Model file for the job. Use its own axes, mm. Face numbers are marked on the shaded views. Coordinates: 2 decimals unless noted, no trailing zeros. Order: outer loops, then holes, each group sorted by start corner. A loop starts at its lowest first (then second) coordinate and runs counter-clockwise, first axis right, second up. Notation, with made-up numbers: (64, -11.5) -> (99, -11.5) arc R13 ccw to (99, -1.5) -> close; hole circle Ø9 at (-8, -17). An arc over 180 degrees is marked (long way). Write item = value, one per line. Start each with the question number.
Q1. Flat gauge pins, fed straight in: pin 1 (8 mm diameter, centred on x = 12.5, y = -11.5, fed in from +Z); pin 2 (10 mm diameter, centred on x = 9.5, z = 22, fed in from +Y); pin 3 (5 mm diameter, centred on x = 11.5, z = 77.5, fed in from +Y); pin 4 (8 mm diameter, centred on y = -5.5, z = 38.5, fed in from -X). Where does each tip first touch, or does it go through?
Q2. Cut at A-A, the plane z = 82.5. List the corners of the cut face in (x, y), plus the area to 3 significant figures.
Q3. Wall check: line 1 (Y direction, x = 5, z = 59.5); line 2 (Z direction, x = -11.5, y = 11); line 3 (X direction, y = 22, z = 76). Give the ranges that are in metal, low to high. Write a range as from..to.
Q4. Cut at B-B, the plane y = 3. List the corners of the cut face in (x, z).
Q5. Cut at D-D, the plane y = -29. List the corners of the cut face in (x, z), plus the area to 3 significant figures.
Q6. Cut at C-C, the plane z = 45.5. List the corners of the cut face in (x, y), plus the area to 3 significant figures.
Q7. Mould opens along Z. For the marked faces 1, 2 and 3 say: +Z half, -Z half, draft (parallel to the pull), parting line (faces both ways), or undercut.
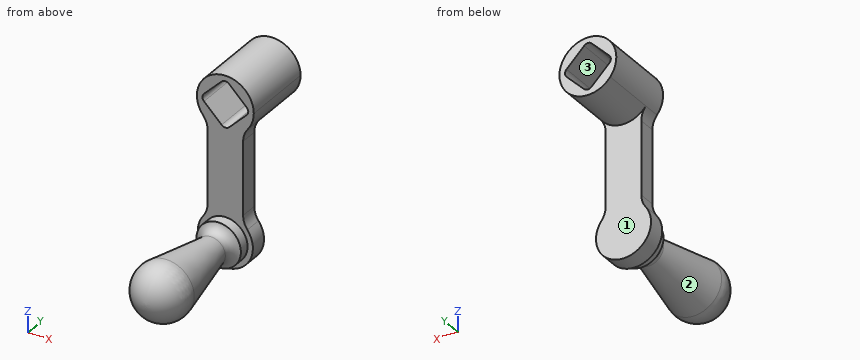
from build123d import *

# Parameters (mm, degrees)
F1_DEPTH = 10
F2_DEPTH = 32


with BuildPart() as f1:
    # F0 (on Front) → F1 (new body)
    with BuildSketch(Plane.XZ):
        with BuildLine():
            ThreePointArc((16, 75), (-5.237229, 90.118579), (-12.571429, 65.102567))
            ThreePointArc((-12.571429, 65.102567), (0, 59), (12.571429, 65.102567))
            ThreePointArc((12.571429, 65.102567), (15.118579, 69.762771), (16, 75))
        make_face()
        with BuildLine():
            Line((2.12132, 87.020815), (12.020815, 77.12132))
            ThreePointArc((12.020815, 77.12132), (12.899495, 75), (12.020815, 72.87868))
            Line((12.020815, 72.87868), (2.12132, 62.979185))
            ThreePointArc((2.12132, 62.979185), (0, 62.100505), (-2.12132, 62.979185))
            Line((-2.12132, 62.979185), (-12.020815, 72.87868))
            ThreePointArc((-12.020815, 72.87868), (-12.899495, 75), (-12.020815, 77.12132))
            Line((-12.020815, 77.12132), (-2.12132, 87.020815))
            ThreePointArc((-2.12132, 87.020815), (0, 87.899495), (2.12132, 87.020815))
        make_face(mode=Mode.SUBTRACT)
        with BuildLine():
            ThreePointArc((-10, 16.5), (-10.6158, 12.705267), (-12.4, 9.3))
            ThreePointArc((-12.4, 9.3), (0, -15.5), (12.4, 9.3))
            ThreePointArc((12.4, 9.3), (10.6158, 12.705267), (10, 16.5))
            Line((10, 16.5), (10, 57.679492))
            ThreePointArc((10, 57.679492), (10.661066, 61.607414), (12.571429, 65.102567))
            ThreePointArc((12.571429, 65.102567), (0, 59), (-12.571429, 65.102567))
            ThreePointArc((-12.571429, 65.102567), (-10.661066, 61.607414), (-10, 57.679492))
            Line((-10, 57.679492), (-10, 16.5))
        make_face()
    extrude(amount=F1_DEPTH)

    # F0 (on Front) → F2 (join)
    with BuildSketch(Plane.XZ):
        with BuildLine():
            ThreePointArc((16, 75), (-5.237229, 90.118579), (-12.571429, 65.102567))
            ThreePointArc((-12.571429, 65.102567), (0, 59), (12.571429, 65.102567))
            ThreePointArc((12.571429, 65.102567), (15.118579, 69.762771), (16, 75))
        make_face()
        with BuildLine():
            Line((2.12132, 87.020815), (12.020815, 77.12132))
            ThreePointArc((12.020815, 77.12132), (12.899495, 75), (12.020815, 72.87868))
            Line((12.020815, 72.87868), (2.12132, 62.979185))
            ThreePointArc((2.12132, 62.979185), (0, 62.100505), (-2.12132, 62.979185))
            Line((-2.12132, 62.979185), (-12.020815, 72.87868))
            ThreePointArc((-12.020815, 72.87868), (-12.899495, 75), (-12.020815, 77.12132))
            Line((-12.020815, 77.12132), (-2.12132, 87.020815))
            ThreePointArc((-2.12132, 87.020815), (0, 87.899495), (2.12132, 87.020815))
        make_face(mode=Mode.SUBTRACT)
    extrude(amount=-F2_DEPTH)

    # F3 (on Right) → F4 (revolve)
    with BuildSketch(Plane.YZ):
        with BuildLine():
            Line((-66, 0), (-10, 0))
            Line((-10, 0), (-10, 12.5))
            Line((-10, 12.5), (-16, 12.5))
            ThreePointArc((-16, 12.5), (-18.595581, 8.930846), (-22.930288, 8.102466))
            Line((-22.930288, 8.102466), (-63.01323, 15.718753))
            ThreePointArc((-63.01323, 15.718753), (-76.203227, 12.324535), (-82, 0))
            Line((-82, 0), (-66, 0))
        make_face()
    revolve(axis=Axis((0, -33, 0), (0, -1, 0)))


solid = f1.part
Here are the results:
q1.pin_1 = 88.37
q1.pin_2 = 0
q1.pin_3 = 32
q1.pin_4 = -10
q2.outline = (-14.13, -10) -> (-6.64, -10) -> (-6.64, 32) -> (-14.13, 32) -> close; (6.64, -10) -> (14.13, -10) -> (14.13, 32) -> (6.64, 32) -> close
q2.area = 629 mm²
q3.line_1 = -10..0
q3.line_2 = 63.88..72.36, 77.64..86.12
q3.line_3 = -15.97..-12.73, 12.73..15.97
q4.outline = (12.57, 65.1) arc R16 ccw to (16, 75) arc R16 ccw (long way) to start; hole (-12.02, 72.88) -> (-2.12, 62.98) arc R3 ccw to (2.12, 62.98) -> (12.02, 72.88) arc R3 ccw to (12.02, 77.12) -> (2.12, 87.02) arc R3 ccw to (-2.12, 87.02) -> (-12.02, 77.12) arc R3 ccw to start
q5.outline = circle Ø18.51 at (0, 0)
q5.area = 269 mm²
q6.outline = (-10, -10) -> (10, -10) -> (10, 0) -> (-10, 0) -> close
q6.area = 200 mm²
q7.face_1 = draft
q7.face_2 = parting line
q7.face_3 = undercut
